For this review, take the finished solid that the model builds, in its own axes (mm). A direction names the side the tool comes from. Give positions to 0.01 mm unless a question says otherwise; leave off trailing zeros. Loops run counter-clockwise (first coordinate to the right, second up) from the corner with the lowest first, then second, coordinate; pieces in that order, holes last. Notation, with made-up numbers: (52, 72.25) - (65, 72.25) arc R20 ccw to (65, 76.25) - close; hole circle Ø11 at (45, 80). An arc over 180 degrees is marked (long way). Use CSV: the item, a comma, the result in double quotes. Start each with the question number.
1. Take a section at D-D on x = 55.5. Give the boundary of the cut face in (y, z), plus the area to 3 significant figures.
2. Wall thickness on line 1 (X direction, y = 1.55, z = -75); line 2 (X direction, y = 0.9, z = 57); line 3 (Z direction, x = -28.5, y = 3.9): over which ranges is each line inside the solid? List them lowest first.
3. Take a section at B-B on z = 38.5. Give the boundary of the cut face in (x, y), plus the area to 3 significant figures.
4. For pin 1 (3.5 mm diameter, centred on y = 3.5, z = 58, fed in from +X); pin 2 (1.6 mm diameter, centred on x = 5.5, y = 3, fed in from +Z); pin 3 (0.9 mm diameter, centred on x = 3.5, y = 2.5, fed in from +Z), all flat-tipped, find the tip position at first contact; note any pin that passes through.
5. Take a section at A-A on x = -4. Give the boundary of the cut face in (y, z).
6. For faces 5 (the flat face through (-64, 3, -1.5)), 6 (the flat face through (50, 3, -72)), 7 (the flat face through (-9, 3, 24)), list the 3-axis set-ups (+Z, -Z, +X, -X, +Y, -Y) from which the entire face can be reached by the end or side of a thin tool; tool diameter is ignored.
7. Take a section at C-C on y = 2.05. State how many separate pieces and enclosed holes the cut face has, plus the area to 3 significant figures.
8. Mouldability with a two-part tool opening along X and no side actions: class faces 1 (the flat face through (-5, 3, 36.485)), 2 (the flat face through (75, 3, -28)), 3 (the flat face through (-72, 3, -50)), 4 (the flat face through (4.5, 3, 64)) as pulls with the +X half, pulls with the -X half, needs draft (parallel to the pull), parting line crosses it, or undercut.
```python
from build123d import *

# Parameters (mm, degrees)
SKETCH1_R           = 1.5
BOSS_EXTRUDE1_DEPTH = 6


with BuildPart() as part:
    # Sketch1 → Boss-Extrude1 (new body)
    with BuildSketch(Plane(origin=(0, 0, 0), x_dir=(1, 0, 0), z_dir=(0, 1, 0))):
        Polygon((-72, 72), (-72, 28), (-66, 28), (-66, 4.5), (-62, 4.5), (-62, 6.5), (-59, 6.5), (-59, 4.5), (-56, 4.5), (-56, 1.5), (-59, 1.5), (-59, -0.5), (-62, -0.5), (-62, 1.5), (-66, 1.5), (-66, -22), (-72, -22), (-72, -72), (-22, -72), (-22, -66), (1.5, -66), (1.5, -62), (-0.5, -62), (-0.5, -59), (1.5, -59), (1.5, -56), (4.5, -56), (4.5, -59), (6.5, -59), (6.5, -62), (4.5, -62), (4.5, -66), (28, -66), (28, -72), (72, -72), (72, -22), (78, -22), (78, 28), (72, 28), (72, 72), (28, 72), (28, 78), (-22, 78), (-22, 72), align=None)
        Polygon((-9, -20.484869039), (7, -20.484869039), (7, -42.484869039), (-9, -42.484869039), (-9, -36.484869039), (-1, -36.484869039), (-1, -26.484869039), (-9, -26.484869039), align=None, mode=Mode.SUBTRACT)
        with Locations(Location((3, 75, 0), (0, 0, 270))):
            Circle(SKETCH1_R, mode=Mode.SUBTRACT)
        with Locations(Location((75, 3, 0), (0, 0, 270))):
            Circle(SKETCH1_R, mode=Mode.SUBTRACT)
    extrude(amount=BOSS_EXTRUDE1_DEPTH)


solid = part.part
```
Check result:
1,outline,"(0, -72) - (6, -72) - (6, 72) - (0, 72) - close"
1,area,"864 mm²"
2,line 1,"x = -22 to 1.5, 4.5 to 28"
2,line 2,"x = -72 to 1.5, 4.5 to 72"
2,line 3,"z = -72 to 72"
3,outline,"(-72, 0) - (-9, 0) - (-9, 6) - (-72, 6) - close; (7, 0) - (72, 0) - (72, 6) - (7, 6) - close"
3,area,"768 mm²"
4,pin 1,"stops at x = 72"
4,pin 2,"stops at z = 66"
4,pin 3,"stops at z = 56"
5,outline,"(0, -78) - (6, -78) - (6, 20.48) - (0, 20.48) - close; (0, 26.48) - (6, 26.48) - (6, 36.48) - (0, 36.48) - close; (0, 42.48) - (6, 42.48) - (6, 66) - (0, 66) - close"
6,face 5,"-X, +Y, -Y"
6,face 6,"-Z, +X, +Y, -Y"
6,face 7,"+Y, -Y"
7,separate pieces,"1"
7,enclosed holes,"3"
7,area,"20,400 mm²"
8,face 1,"undercut"
8,face 2,"needs draft"
8,face 3,"pulls with the -X half"
8,face 4,"undercut"
